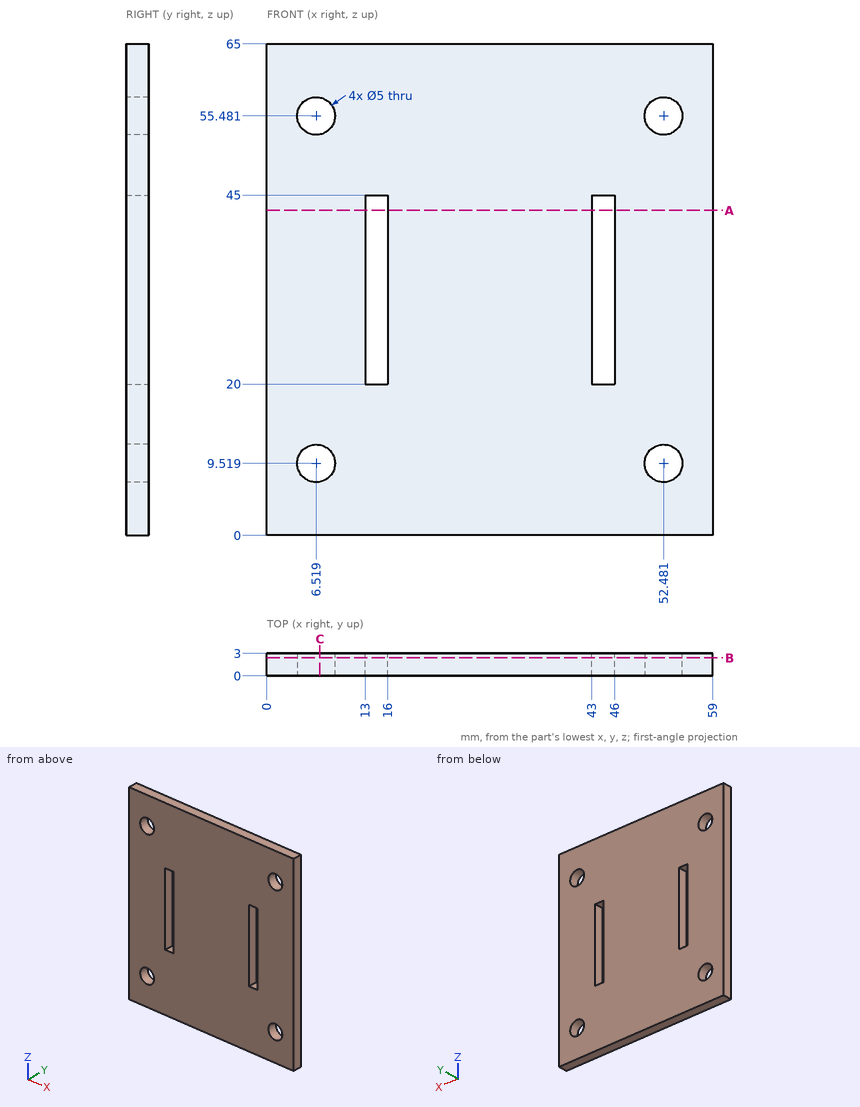
Drawing for the job (mm, zero at the part's lowest x, y, z). Round coordinates to 2 decimals unless told otherwise and drop trailing zeros. Write each loop counter-clockwise with the first axis right and the second up, starting at its lowest first coordinate (ties: lowest second). Pieces come first, ordered by that corner, then holes. Notation, with made-up numbers: M -31,29 L 9,29 A15 ccw 9,35 Z; hole C 36,71 d6. An arc over 180 degrees is marked long. Answer in a Markdown table with one row per item.
1. Saw through at B-B (y = 2.4). List the corners of the cut face in (x, z).
Geometry check:
| item | result |
|---|---|
| outline | M 0,0 L 59,0 L 59,65 L 0,65 Z; hole C 6.52,9.52 d5; hole C 6.52,55.48 d5; hole M 13,20 L 16,20 L 16,45 L 13,45 Z; hole M 43,20 L 46,20 L 46,45 L 43,45 Z; hole C 52.48,9.52 d5; hole C 52.48,55.48 d5 |
2. Probe L1, parallel to X at y = 0.25, z = 42; L2, parallel to Z at x = 4.5, y = 1.6; L3, parallel to Z at x = 54, y = 1.7. List the from-to ranges inside material, lowest first. Write a range as [from, to].
Geometry check:
| item | result |
|---|---|
| L1 | [0, 13], [16, 43], [46, 59] |
| L2 | [0, 8.04], [10.99, 54.01], [56.96, 65] |
| L3 | [0, 7.53], [11.5, 53.5], [57.47, 65] |
3. Saw through at C-C (x = 7). List the corners of the cut face in (y, z).
Geometry check:
| item | result |
|---|---|
| outline | M 0,0 L 3,0 L 3,7.07 L 0,7.07 Z; M 0,11.97 L 3,11.97 L 3,53.03 L 0,53.03 Z; M 0,57.93 L 3,57.93 L 3,65 L 0,65 Z |
4. Flat gauge pin, fed straight in: P1, Ø3, axis at x = 52.48, z = 9.52, coming from the -Y side. Where does the tip first touch, or does it go through?
Geometry check:
| item | result |
|---|---|
| P1 | through |
5. Saw through at A-A (z = 43). List the corners of the cut face in (x, y).
Geometry check:
| item | result |
|---|---|
| outline | M 0,0 L 13,0 L 13,3 L 0,3 Z; M 16,0 L 43,0 L 43,3 L 16,3 Z; M 46,0 L 59,0 L 59,3 L 46,3 Z |
